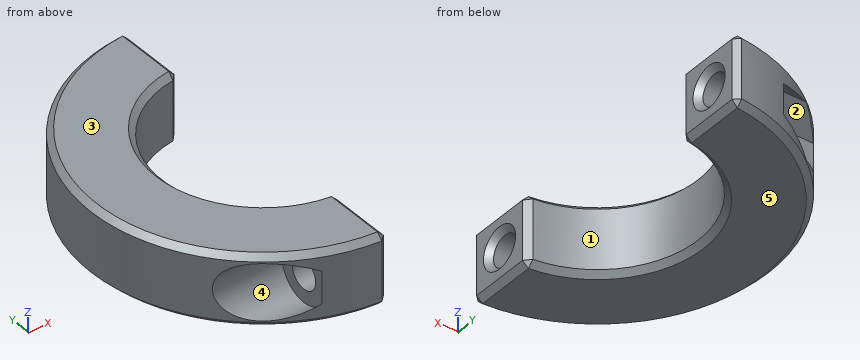
```python
from build123d import *

# Parameters (mm, degrees)
PAD_DEPTH       = 10
SKETCH001_R     = 2.15
POCKET_DEPTH    = 23.236509
SKETCH002_R     = 4
POCKET001_DEPTH = 15.236509
SKETCH003_R     = 2.15
POCKET002_DEPTH = 23.236509
POCKET003_DEPTH = 15.236509
CHAMFER_SIZE    = 0.8


with BuildPart() as part:
    # Sketch → Pad (new body)
    with BuildSketch(Plane.XY):
        with BuildLine():
            Line((-1, 14.214869), (-1, 24.214869))
            ThreePointArc((-1, 24.214869), (-24.235509, 0), (-1, -24.214869))
            Line((-1, -24.214869), (-1, -14.214869))
            ThreePointArc((-1, 14.214869), (-14.25, 0), (-1, -14.214869))
        make_face()
    extrude(amount=PAD_DEPTH)

    # Sketch001 (on Face3 of Pad) → Pocket (cut, through all)
    with BuildSketch(Plane.YZ.offset(-1)):
        with Locations((-19.214869, 5)):
            Circle(SKETCH001_R)
    extrude(amount=-POCKET_DEPTH, mode=Mode.SUBTRACT)

    # Sketch002 (on DatumPlane) → Pocket001 (cut, through all)
    with BuildSketch(Plane(origin=(-9, -19.214869, 5), x_dir=(0, -1, 0), z_dir=(-1, 0, 0))):
        Circle(SKETCH002_R)
    extrude(amount=POCKET001_DEPTH, mode=Mode.SUBTRACT)

    # Sketch003 (on Face1 of Pocket001) → Pocket002 (cut, through all)
    with BuildSketch(Plane.YZ.offset(-1)):
        with Locations((19.214869, 5)):
            Circle(SKETCH003_R)
    extrude(amount=-POCKET002_DEPTH, mode=Mode.SUBTRACT)

    # Sketch004 (on DatumPlane) → Pocket003 (cut, through all)
    with BuildSketch(Plane(origin=(-9, -19.214869, 5), x_dir=(0, -1, 0), z_dir=(-1, 0, 0))):
        Polygon((-41.929738, 2.020726), (-41.929738, -2.020726), (-38.429738, -4.041452), (-34.929738, -2.020726), (-34.929738, 2.020726), (-38.429738, 4.041452), align=None)
    extrude(amount=POCKET003_DEPTH, mode=Mode.SUBTRACT)

    # Chamfer
    chamfer_edges = [part.edges().sort_by_distance(p)[0] for p in [
        (-1, 19.214869, 10),
        (-24.235509, 0, 10),
        (-1, -19.214869, 10),
        (-14.25, 0, 10),
        (-1, 19.214869, 0),
        (-24.235509, 0, 0),
        (-1, -19.214869, 0),
        (-14.25, 0, 0),
        (-1, 14.214869, 5),
        (-1, 24.214869, 5),
        (-1, 17.064869, 5),
        (-1, -24.214869, 5),
        (-1, -14.214869, 5),
        (-1, -21.364869, 5),
    ]]
    chamfer(chamfer_edges, length=CHAMFER_SIZE)


solid = part.part
```
Verification items for the finished model (mm, model axes). Face numbers are marked on the shaded views. A direction names the side the tool comes from. Give positions to 0.01 mm unless a question says otherwise; leave off trailing zeros. Write each loop counter-clockwise with the first axis right and the second up, starting at its lowest first coordinate (ties: lowest second). Pieces come first, ordered by that corner, then holes. Notation, with made-up numbers: (-11.75, 19.5) - (-7.75, 19.5) arc R20 cw to (-7.75, 39.5) - close; hole circle Ø6 at (-16, -33.5). An arc over 180 degrees is marked (long way). Put each result on its own line as item: value.
Q1. Depth check by flat-ended pin: P1, Ø4, axis at y = 19.21, z = 5, coming from the +X side; P2, Ø5, axis at y = 2.5, z = 5.5, coming from the +X side; P3, Ø1, axis at x = -12, z = 3, coming from the -Y side; P4, Ø12, axis at x = -19.5, y = -17.5, coming from the +Z side. Enter the tip coordinate at first touch or a pass-through.
Result:
P1: through
P2: x = -13.34
P3: y = -16.09
P4: z = 10
Q2. Scan lines: probe 1 along Y at (x, z) = (-5, 6.5); probe 2 along Y at (x, z) = (-9.75, 7.5) (3 decimals); probe 3 along Y at (x, z) = (-8, 5.75). Record each from-to range of solid material in increasing order. Write a range as from..to.
Result:
probe 1: -23.71..-20.76, -17.67..-13.34, 13.34..17.67, 20.76..23.71
probe 2: -16.092..-10.392, 10.392..16.545, 21.885..22.188
probe 3: -22.88..-21.23, -17.2..-11.79, 11.79..17.2, 21.23..22.88
Q3. Section check B-B on x = -6.75. Count the separate pieces of the cut face and the enclosed holes in it, and give its area (3 significant figures).
Result:
separate pieces: 2
enclosed holes: 2
area: 183 mm2
Q4. Mould release check, pull along Z, two halves, no side actions. Record for the marked faces 1, 2 and 3: released by +Z, released by -Z, zero draft, split by the parting line, or undercut.
Result:
face 1: zero draft
face 2: undercut
face 3: released by +Z
Q5. Section check A-A on z = 5. Record the cut outline in (x, y), and give its area (3 significant figures).
Result:
outline: (-18.86, -15.21) - (-9, -15.21) - (-9, -17.06) - (-1.8, -17.06) - (-1, -16.26) - (-1, -15.01) - (-1.8, -14.14) arc R14.25 cw to (-1.8, 14.14) - (-1, 15.01) - (-1, 16.26) - (-1.8, 17.06) - (-9, 17.06) - (-9, 15.71) - (-18.45, 15.71) arc R24.24 ccw to start; (-9, -22.5) arc R24.24 ccw to (-1.8, -24.17) - (-1, -23.41) - (-1, -22.16) - (-1.8, -21.36) - (-9, -21.36) - close; (-9, 21.36) - (-1.8, 21.36) - (-1, 22.16) - (-1, 23.41) - (-1.8, 24.17) arc R24.24 ccw to (-9, 22.5) - close
area: 432 mm2
Q6. Set-up check for the marked faces 4 and 5: record each of +Z, -Z, +X, -X, +Y, -Y from which the full face is reachable in a straight line by a thin tool's end or side.
Result:
face 4: -X
face 5: -Z, +X, -X, +Y, -Y
